```python
from build123d import *

# Parameters (mm, degrees)
F0_R     = 12.7
F1_DEPTH = 28.575
F2_R     = 11.1125
F3_DEPTH = 12.7
F5_DEPTH = 25.4
F6_R     = 3.96875
F7_DEPTH = 23.242
F9_DEPTH = 23.242


with BuildPart() as f1:
    # F0 (on Right) → F1 (new body)
    with BuildSketch(Plane.YZ):
        Circle(F0_R)
    extrude(amount=F1_DEPTH)

    # F2 (on face) → F3 (join)
    with BuildSketch(Plane(origin=(0, 0, 0), x_dir=(0, -1, 0), z_dir=(-1, 0, 0))):
        Circle(F2_R)
    extrude(amount=F3_DEPTH)

    # F4 (on face) → F5 (cut)
    with BuildSketch(Plane.YZ.offset(28.575)):
        with BuildLine():
            Line((-10.541, 7.0835950618), (-10.541, 10.541))
            Line((-10.541, 10.541), (-7.0835950618, 10.541))
            ThreePointArc((-7.0835950618, 10.541), (0, 12.7), (7.0835950618, 10.541))
            Line((7.0835950618, 10.541), (14.6175222471, 10.541))
            Line((14.6175222471, 10.541), (14.6175222471, 13.3875589818))
            Line((14.6175222471, 13.3875589818), (-14.6175222471, 13.3875589818))
            Line((-14.6175222471, 13.3875589818), (-14.6175222471, -13.3875589818))
            Line((-14.6175222471, -13.3875589818), (14.6175222471, -13.3875589818))
            Line((14.6175222471, -13.3875589818), (14.6175222471, -10.541))
            Line((14.6175222471, -10.541), (7.0835950618, -10.541))
            ThreePointArc((7.0835950618, -10.541), (0, -12.7), (-7.0835950618, -10.541))
            Line((-7.0835950618, -10.541), (-10.541, -10.541))
            Line((-10.541, -10.541), (-10.541, -7.0835950618))
            ThreePointArc((-10.541, -7.0835950618), (-12.7, 0), (-10.541, 7.0835950618))
        make_face()
        with BuildLine():
            ThreePointArc((7.0835950618, 10.541), (0, 12.7), (-7.0835950618, 10.541))
            Line((-7.0835950618, 10.541), (7.0835950618, 10.541))
        make_face()
        with BuildLine():
            Line((-10.541, -7.0835950618), (-10.541, 7.0835950618))
            ThreePointArc((-10.541, 7.0835950618), (-12.7, 0), (-10.541, -7.0835950618))
        make_face()
        with BuildLine():
            Line((7.0835950618, -10.541), (-7.0835950618, -10.541))
            ThreePointArc((-7.0835950618, -10.541), (0, -12.7), (7.0835950618, -10.541))
        make_face()
    extrude(amount=-F5_DEPTH, mode=Mode.SUBTRACT)

    # F6 (on face) → F7 (cut, through all)
    with BuildSketch(Plane.XY.offset(10.541)):
        with Locations((22.225, 0)):
            Circle(F6_R)
    extrude(amount=-F7_DEPTH, mode=Mode.SUBTRACT)

    # F8 (on face) → F9 (cut, through all)
    with BuildSketch(Plane.XY.offset(10.541)):
        with BuildLine():
            ThreePointArc((32.766, 0), (29.6786125805, -7.4536125805), (22.225, -10.541))
            Line((22.225, -10.541), (22.225, -14.2959095994))
            ThreePointArc((22.225, -14.2959095994), (32.333734621, -10.108734621), (36.5209095994, 0))
            Line((36.5209095994, 0), (32.766, 0))
        make_face()
    extrude(amount=-F9_DEPTH, mode=Mode.SUBTRACT)


solid = f1.part
```
Model file for the job. Use its own axes, mm. A direction names the side the tool comes from. Coordinates: 2 decimals unless noted, no trailing zeros. Write each loop counter-clockwise with the first axis right and the second up, starting at its lowest first coordinate (ties: lowest second). Pieces come first, ordered by that corner, then holes. Notation, with made-up numbers: (-24.75, 42) - (28.25, 42) arc R23 ccw to (28.25, 63) - close; hole circle Ø8 at (49.25, -25). An arc over 180 degrees is marked (long way). One line per question, with ' | ' between items. Start each with the question number.
Q1. Cut at A-A, the plane z = 0. List the corners of the cut face in (x, y) (1 decimal).
Q2. Cut at B-B, the plane y = 0. List the corners of the cut face in (x, z) (1 decimal).
Q3. Pull direction X, two halves, no side cores. Call faces 1 (the face through (-12.7, 0, 0)), 2 (the face through (18.26, 0.17, 0.15)), 3 (the face through (16, 0, -10.541)): pulls with the +X half, pulls with the -X half, needs draft (parallel to the pull), parting line crosses it, or undercut.
Q4. 3-axis set-ups, long thin cutter, end or side, ignore diameter. For faces 4 (the face through (0, 0.88, -11.23)), 5 (the face through (3.175, 0, -11)), 6 (the face through (3.175, 0, 11)), 7 (the face through (3.175, -11, 0)): which of +Z, -Z, +X, -X, +Y, -Y reach the whole face in a straight line?
Q5. Cut at C-C, the plane x = 20.5. List the corners of the cut face in (y, z), then the cut area to 3 significant figures.
Q6. Cut at D-D, the plane y = -3. List the corners of the cut face in (x, z) (3 decimals), then the cut area to 3 significant figures.
Q7. Drill centre lines: line 1 (Z direction, x = 5, y = 4); line 2 (Y direction, x = 22.5, z = -8.75); line 3 (X direction, y = 2.25, z = 9.75) (3 decimals). Where is each one in solid material? Low to high. Write a range as [from, to].
Q8. Pin check, flat tips, straight feed: pin 1 (1 mm diameter, centred on x = 6, y = 8, fed in from +Z); pin 2 (2.5 mm diameter, centred on y = -11, z = 0, fed in from +X); pin 3 (1.1 mm diameter, centred on y = -0.5, z = 11.5, fed in from +X) (3 decimals). Stop position of each tip, or through.
Answer below:
1) outline: (-12.7, -11.1) - (0, -11.1) - (0, -12.7) - (3.2, -12.7) - (3.2, -10.5) - (22.2, -10.5) arc R10.5 ccw to (28.6, -8.4) - (28.6, 12.7) - (0, 12.7) - (0, 11.1) - (-12.7, 11.1) - close; hole circle Ø7.9 at (22.2, 0)
2) outline: (-12.7, -11.1) - (0, -11.1) - (0, -12.7) - (3.2, -12.7) - (3.2, -10.5) - (18.3, -10.5) - (18.3, 10.5) - (3.2, 10.5) - (3.2, 12.7) - (0, 12.7) - (0, 11.1) - (-12.7, 11.1) - close; (26.2, -10.5) - (28.6, -10.5) - (28.6, 10.5) - (26.2, 10.5) - close
3) face 1: pulls with the -X half | face 2: undercut | face 3: needs draft
4) face 4: -X | face 5: -Z, +X, +Y, -Y | face 6: +Z, +X, +Y, -Y | face 7: +Z, -Z, +X, -Y
5) outline: (-10.54, -7.08) arc R12.7 ccw to (-7.08, -10.54) - (-3.57, -10.54) - (-3.57, 10.54) - (-7.08, 10.54) arc R12.7 ccw to (-10.54, 7.08) - close; (3.57, -10.54) - (7.08, -10.54) arc R12.7 ccw to (7.08, 10.54) - (3.57, 10.54) - close | area: 294 mm^2
6) outline: (-12.7, -10.7) - (0, -10.7) - (0, -12.341) - (3.175, -12.341) - (3.175, -10.541) - (19.627, -10.541) - (19.627, 10.541) - (3.175, 10.541) - (3.175, 12.341) - (0, 12.341) - (0, 10.7) - (-12.7, 10.7) - close; (24.823, -10.541) - (28.575, -10.541) - (28.575, 10.541) - (24.823, 10.541) - close | area: 776 mm^2
7) line 1: [-10.54, 10.54] | line 2: [-9.2, -3.96], [3.96, 9.2] | line 3: [-12.7, 18.956], [25.494, 28.575]
8) pin 1: z = 10.25 | pin 2: x = 26.23 | pin 3: x = 3.175
